Geometry check sheet. Reference: the model listing, model coordinates, mm. Face numbers are marked on the shaded views. Round coordinates to 2 decimals unless told otherwise and drop trailing zeros. Order: outer loops, then holes, each group sorted by start corner. A loop starts at its lowest first (then second) coordinate and runs counter-clockwise, first axis right, second up.
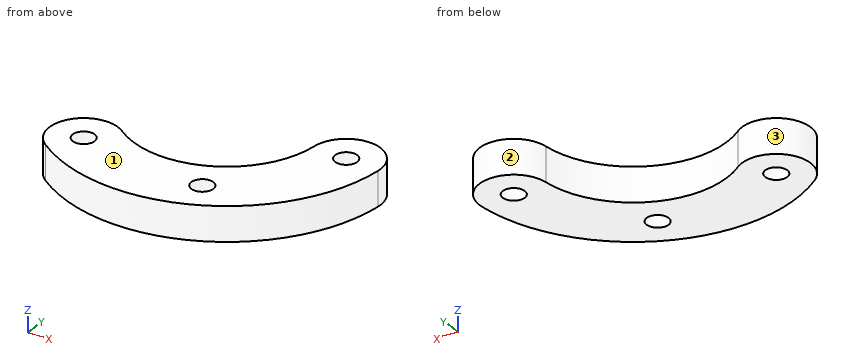
```python
from build123d import *

# Parameters (mm, degrees)
SKETCH_1_R      = 1.6
EXTRUDE_1_DEPTH = 5


with BuildPart() as part:
    # 草图1 → 凸台-拉伸1 (new body)
    with BuildSketch(Plane.XY):
        with BuildLine():
            ThreePointArc((-3.016005594, -3.963654581), (20.711469165, -6.788370191), (34.699500163, 12.584473316))
            ThreePointArc((34.699500163, 12.584473316), (30.205119406, 18.007962633), (24.781630088, 13.513581877))
            ThreePointArc((24.781630088, 13.513581877), (16.709135129, 2.333510745), (3.016005594, 3.963654581))
            ThreePointArc((3.016005594, 3.963654581), (-3.963654581, 3.016005594), (-3.016005594, -3.963654581))
        make_face()
        Circle(SKETCH_1_R, mode=Mode.SUBTRACT)
        with Locations((29.740565125, 13.049027596)):
            Circle(SKETCH_1_R, mode=Mode.SUBTRACT)
        with Locations((18.710302147, -2.227429723)):
            Circle(SKETCH_1_R, mode=Mode.SUBTRACT)
    extrude(amount=EXTRUDE_1_DEPTH)


solid = part.part
```
(1) Draft check along X on the marked faces 1, 2 and 3. Enter one of: released by +X, released by -X, zero draft, split by the parting line, or undercut.
Returned:
face 1: zero draft
face 2: split by the parting line
face 3: undercut
(2) Sectioned sample at C-C, the plane z = 2.4. Record the cut outline in (x, y).
Returned:
outline: (-3.02, -3.96) arc R23.55 ccw to (34.7, 12.58) arc R4.98 ccw to (24.78, 13.51) arc R13.59 cw to (3.02, 3.96) arc R4.98 ccw to start; hole circle Ø3.2 at (0, 0); hole circle Ø3.2 at (18.71, -2.23); hole circle Ø3.2 at (29.74, 13.05)
(3) Depth check by flat-ended pin: P1, Ø2.5, axis at x = 18.71, y = -2.23, coming from the +Z side; P2, Ø1, axis at x = 13.5, z = 1, coming from the -Y side; P3, Ø1.5, axis at y = 4, z = 1, coming from the +X side; P4, Ø3, axis at y = -4.5, z = 2.5, coming from the +X side. Enter the tip coordinate at first touch or a pass-through.
Returned:
P1: passes through
P2: stops at y = -8.71
P3: stops at x = 32.56
P4: stops at x = 26.7
(4) Sectioned sample at D-D, the plane y = 6. Record the cut outline in (x, z), and give its area (3 significant figures).
Returned:
outline: (21.62, 0) - (33.1, 0) - (33.1, 5) - (21.62, 5) - close
area: 57.4 mm2
(5) Sectioned sample at A-A, the plane x = 0. Record the cut outline in (y, z), and give its area (3 significant figures).
Returned:
outline: (-5.91, 0) - (-1.6, 0) - (-1.6, 5) - (-5.91, 5) - close; (1.6, 0) - (4.98, 0) - (4.98, 5) - (1.6, 5) - close
area: 38.5 mm2
(6) Material ranges on line 1 (Y direction, x = 20, z = 0.6); line 2 (X direction, y = 12.25, z = 1.2); line 3 (X direction, y = 0.75, z = 2.2), recorded low to high.
Returned:
line 1: y = -7.09 to -3.17, -1.28 to 4.38
line 2: x = 24.6 to 28.35, 31.13 to 34.67
line 3: x = -4.92 to -1.41, 1.41 to 30.17
(7) Sectioned sample at B-B, the plane y = 0. Record the cut outline in (x, z), and give its area (3 significant figures).
Returned:
outline: (-4.98, 0) - (-1.6, 0) - (-1.6, 5) - (-4.98, 5) - close; (1.6, 0) - (29.59, 0) - (29.59, 5) - (1.6, 5) - close
area: 157 mm2
